```python
from build123d import *

# Parameters (mm, degrees)
SKETCH_2_W                       = 60
SKETCH_2_H                       = 14.8
CUT_EXTRUDE_1_DEPTH              = 88.258695842
FILLET_2_R                       = 2
PATTERN_CIRCULAR_1_COUNT         = 8
FILLET_2_OF_PATTERN_CIRCULAR_1_R = 2


with BuildPart() as part:
    # Эскиз2 → Повернуть1 (revolve)
    with BuildSketch(Plane(origin=(0, 0, 0), x_dir=(0, 0, -1), z_dir=(1, 0, 0)), mode=Mode.PRIVATE) as revolve_1_sk:
        with Locations((30, 37.4)):
            Rectangle(SKETCH_2_W, SKETCH_2_H)
    revolve(revolve_1_sk.sketch.rotate(Axis((0, 0, 0), (0, 0, -1)), 90), axis=Axis((0, 0, 0), (0, 0, -1)))

    # Эскиз4 → Вырез-Вытянуть1 (cut, through all)
    with BuildSketch(Plane.XY):
        with BuildLine():
            Line((-5.8, 37.554760018), (-5.8, 44.422967033))
            ThreePointArc((-5.8, 44.422967033), (-11.571918734, 43.279679953), (-17.14421777, 41.389803057))
            Line((-17.14421777, 41.389803057), (-14.54197043, 35.107422235))
            ThreePointArc((-14.54197043, 35.107422235), (-10.244330422, 36.5930826), (-5.8, 37.554760018))
        make_face()
        with BuildLine():
            Line((5.8, 37.554760018), (5.8, 44.422967033))
            ThreePointArc((5.8, 44.422967033), (11.571918734, 43.279679953), (17.14421777, 41.389803057))
            Line((17.14421777, 41.389803057), (14.54197043, 35.107422235))
            ThreePointArc((14.54197043, 35.107422235), (10.244330422, 36.5930826), (5.8, 37.554760018))
        make_face()
    cut_extrude_1 = extrude(amount=-CUT_EXTRUDE_1_DEPTH, mode=Mode.SUBTRACT)

    # Скругление2
    fillet_2_edges = [part.edges().sort_by_distance(p)[0] for p in [
        (-5.8, 37.554760018, -30),
        (5.8, 37.554760018, -30),
    ]]
    fillet(fillet_2_edges, radius=FILLET_2_R)

    # Круговой массив1: Вырез-Вытянуть1 ×8 about axis
    pattern_circular_1_axis = Axis((0, 0, 0), (0, 0, 1))
    for i in range(1, PATTERN_CIRCULAR_1_COUNT):
        add(cut_extrude_1.rotate(pattern_circular_1_axis, i * 360 / PATTERN_CIRCULAR_1_COUNT), mode=Mode.SUBTRACT)

    # Скругление2 of Круговой массив1
    fillet_2_of_pattern_circular_1_edges = [part.edges().sort_by_distance(p)[0] for p in [
        (-30.656444805, 22.454006144, -30),
        (-22.454006144, 30.656444805, -30),
        (-37.554760018, -5.8, -30),
        (-37.554760018, 5.8, -30),
        (-22.454006144, -30.656444805, -30),
        (-30.656444805, -22.454006144, -30),
        (5.8, -37.554760018, -30),
        (-5.8, -37.554760018, -30),
        (30.656444805, -22.454006144, -30),
        (22.454006144, -30.656444805, -30),
        (37.554760018, 5.8, -30),
        (37.554760018, -5.8, -30),
        (22.454006144, 30.656444805, -30),
        (30.656444805, 22.454006144, -30),
    ]]
    fillet(fillet_2_of_pattern_circular_1_edges, radius=FILLET_2_OF_PATTERN_CIRCULAR_1_R)


solid = part.part
```
Build history of the part. All positions in model axes, mm. A direction names the side the tool comes from. Round coordinates to 2 decimals unless told otherwise and drop trailing zeros. Write each loop counter-clockwise with the first axis right and the second up, starting at its lowest first coordinate (ties: lowest second). Pieces come first, ordered by that corner, then holes.
1) 3-axis set-ups, long thin cutter, end or side, ignore diameter. For faces 1 (the flat face through (25.45, -33.65, -29.58)), 2 (the flat face through (-5.8, 42, -30)), 3 (the flat face through (42, 5.8, -30)): which of +Z, -Z, +X, -X, +Y, -Y reach the whole face in a straight line?
2) Band-saw the part on A-A, the plane y = 0. List the corners of the cut face in (x, z).
3) Mould opens along Y. For faces 4 (the flat face through (25.45, 33.65, -29.58)), 5 (the flat face through (7, -30, 0)), 6 (the flat face through (-33.65, 25.45, -29.58)) say: +Y half, -Y half, draft (parallel to the pull), parting line (faces both ways), or undercut.
4) Band-saw the part on C-C, the plane y = 33. List the corners of the cut face in (x, z), and give its area (3 significant figures).
5) Pin check, flat tips, straight feed: pin 1 (3 mm diameter, centred on x = -27, z = -37, fed in from -Y); pin 2 (4 mm diameter, centred on y = -42, z = -15.5, fed in from -X); pin 3 (1 mm diameter, centred on y = 28, z = -39, fed in from +X); pin 4 (12 mm diameter, centred on x = -1.5, y = 18.5, fed in from -Z). Stop position of each tip, or through.
6) Drill centre lines: probe 1 along Y at (x, z) = (0, -21); probe 2 along X at (y, z) = (32, -36.5). Where is each one in solid material? Low to high.
Ans:
1. face 1: +Z, -Z, -Y
1. face 2: +Z, -Z, -X, +Y
1. face 3: +Z, -Z, +X, +Y
2. outline: (-44.8, -60) - (-30, -60) - (-30, 0) - (-44.8, 0) - close; (30, -60) - (44.8, -60) - (44.8, 0) - (30, 0) - close
3. face 4: +Y half
3. face 5: draft
3. face 6: undercut
4. outline: (-30.3, -60) - (-24.8, -60) - (-24.8, 0) - (-30.3, 0) - close; (-18.84, -60) - (18.84, -60) - (18.84, 0) - (-18.84, 0) - close; (24.8, -60) - (30.3, -60) - (30.3, 0) - (24.8, 0) - close
4. area: 2,920 mm2
5. pin 1: stops at y = -35.51
5. pin 2: stops at x = -5.8
5. pin 3: stops at x = 35.37
5. pin 4: passes through
6. probe 1: y = -44.8 to -30, 30 to 44.8
6. probe 2: x = -31.35 to -23.8, -20.49 to 20.49, 23.8 to 31.35
